```python
from build123d import *

# Parameters (mm, degrees)
CHAMFER1_SIZE               = 1
SKETCH3_R                   = 4.7625
BOSS_EXTRUDE1_DEPTH         = 17
CHAMFER2_SIZE               = 1
F_1_4_28_TAPPED_HOLE1_D     = 5.4102
F_1_4_28_TAPPED_HOLE1_DEPTH = 15.42
F_1_4_28_TAPPED_HOLE1_TIP   = 1.625388061


with BuildPart() as part:
    # Sketch1 → Revolve1 (revolve)
    with BuildSketch(Plane(origin=(0, 0, 0), x_dir=(0, 0, -1), z_dir=(1, 0, 0))):
        Polygon((-8, 8.5), (-14, 7.9375), (-35, 7.9375), (-57, 7.9375), (-57, 0), (57, 0), (57, 7.9375), (35, 7.9375), (14, 7.9375), (8, 8.5), (8, 8.05), (7, 8.05), (7, 8.5), (-7, 8.5), (-7, 8.05), (-8, 8.05), align=None)
    revolve(axis=Axis((0, 0, 83.804844788), (0, 0, -1)))

    # Chamfer1
    chamfer1_edges = [part.edges().sort_by_distance(p)[0] for p in [
        (0, -7.9375, 57),
        (0, -7.9375, -57),
    ]]
    chamfer(chamfer1_edges, length=CHAMFER1_SIZE)

    # Sketch3 → Boss-Extrude1 (add)
    with BuildSketch(Plane.XY.offset(-57)):
        Circle(SKETCH3_R)
    extrude(amount=-BOSS_EXTRUDE1_DEPTH)

    # Chamfer2
    chamfer2_edges = [part.edges().sort_by_distance(p)[0] for p in [
        (-4.7625, 0, -74),
    ]]
    chamfer(chamfer2_edges, length=CHAMFER2_SIZE)

    # 1/4-28 Tapped Hole1
    with Locations(Plane.XY.offset(57)):
        with Locations((0, 0)):
            Hole(F_1_4_28_TAPPED_HOLE1_D / 2, depth=F_1_4_28_TAPPED_HOLE1_DEPTH)
            with Locations((0, 0, -(F_1_4_28_TAPPED_HOLE1_DEPTH + F_1_4_28_TAPPED_HOLE1_TIP / 2))):  # 118° drill point
                Cone(0, F_1_4_28_TAPPED_HOLE1_D / 2, F_1_4_28_TAPPED_HOLE1_TIP, mode=Mode.SUBTRACT)


solid = part.part
```
CAD build for the part. Positions are in the model's coordinates, mm. A direction names the side the tool comes from. Coordinates: 2 decimals unless noted, no trailing zeros. Order: outer loops, then holes, each group sorted by start corner. A loop starts at its lowest first (then second) coordinate and runs counter-clockwise, first axis right, second up. Notation, with made-up numbers: (67, 79.5) -> (89, 79.5) arc R12 cw to (89, 86.5) -> close; hole circle Ø10 at (-13.75, 10). An arc over 180 degrees is marked (long way). Use one line per item in the form item = value. Start each with the question number.
1) Drop flat-ended pins along their axis: pin 1 (8 mm diameter, centred on y = 6, z = -59, fed in from -X); pin 2 (2 mm diameter, centred on x = 4, z = -51.5, fed in from -Y); pin 3 (8 mm diameter, centred on x = 0.5, z = -52.5, fed in from -Y). Give the stop position or say it passes through.
2) Band-saw the part on A-A on z = 43. Give the cut face in (x, y) (1 decimal).
3) Tool access for faces 1 (the cylindrical face through (-7.75, -1.72, 35.29)), 2 (the flat face through (0, 3, 57)), 3 (the flat face through (2, -5, -57)), 4 (the cylindrical face through (2.418, 7.678, 7.507)): list every direction of +Z, -Z, +X, -X, +Y, -Y with a clear straight run to the whole face (end or side of a thin tool).
4) Pull direction Y, two halves, no side cores. Call faces 5 (the cylindrical face through (-3.78, -2.9, -64.89)), 6 (the flat face through (0, 0, -74)), 7 (the cylindrical face through (-2.58, 0.81, 49.18)): +Y half, -Y half, draft (parallel to the pull), parting line (faces both ways), or undercut.
5) Drill centre lines: L1, parallel to X at y = 0, z = 45; L2, parallel to Y at x = -0.5, z = 31.5; L3, parallel to Z at x = -5, y = -1.25. Where is each one in solid material? Low to high. Write a range as [from, to].
Entries:
q1.pin_1 = -7.19
q1.pin_2 = -7.35
q1.pin_3 = -7.94
q2.outline = circle Ø15.9 at (0, 0); hole circle Ø5.4 at (0, 0)
q3.face_1 = +Z
q3.face_2 = +Z, +X, -X, +Y, -Y
q3.face_3 = -Z
q3.face_4 = none
q4.face_5 = parting line
q4.face_6 = draft
q4.face_7 = undercut
q5.L1 = [-7.94, -2.71], [2.71, 7.94]
q5.L2 = [-7.92, 7.92]
q5.L3 = [-57, 57]
